Work out the finished part from the listing and answer in its coordinate system (mm). A direction names the side the tool comes from. Coordinates: 2 decimals unless noted, no trailing zeros. Write each loop counter-clockwise with the first axis right and the second up, starting at its lowest first coordinate (ties: lowest second). Pieces come first, ordered by that corner, then holes. Notation, with made-up numbers: M 54,-32.75 L 106,-32.75 A35 ccw 106,5.25 Z; hole C -27.5,33 d8. An arc over 180 degrees is marked long. Answer as CSV lines item,"result". Start each with the question number.
(1) For faces 4 (the cylindrical face through (13.62, 2.46, 12.06)), 5 (the flat face through (-40, 2, 1)), determine the directions among +Z, -Z, +X, -X, +Y, -Y from which every point of the face is accessible in a straight line to the end or side of a thin tool.
(2) A flat-ended cylindrical pin translates along its axis: P1, Ø2.5, axis at x = 25, z = -34, coming from the -Y side. Find the tip coordinate at first contact, or state that the pin passes through.
(3) Find the intervals of material crossed by L1, parallel to Z at x = 25, y = 3.25; L2, parallel to X at y = 3.1, z = 34; L3, parallel to Z at x = -4, y = 3.7, in increasing order. Write a range as [from, to].
(4) A cutting plane is placed at C-C on y = 2.6. Give the vertices of the cut face in (x, z).
(5) The mould has two halves that part along Z. Classify faces 1 (the flat face through (-5, 2, 39)), 2 (the flat face through (-5, 2, 13.621)), 3 (the cylindrical face through (-39.14, 2.54, -38.1)): released by +Z, released by -Z, zero draft, split by the parting line, or undercut.
(6) A cutting plane is placed at D-D on x = -7. Give the vertices of the cut face in (y, z), then the cut area to 3 significant figures.
(7) A cutting plane is placed at B-B on z = 0. Give the vertices of the cut face in (x, y), then the cut area to 3 significant figures.
(8) A cutting plane is placed at A-A on x = 25. Give the vertices of the cut face in (y, z), then the cut area to 3 significant figures.
from build123d import *

# Parameters (mm, degrees)
SKETCH1_W           = 70
SKETCH1_H           = 78
SKETCH1_R           = 2.25
BOSS_EXTRUDE1_DEPTH = 5
FILLET1_R           = 3


with BuildPart() as part:
    # Sketch1 → Boss-Extrude1 (new body)
    with BuildSketch(Plane(origin=(0, 0, 0), x_dir=(1, 0, 0), z_dir=(0, 1, 0))):
        with Locations((-5, 0)):
            Rectangle(SKETCH1_W, SKETCH1_H)
        with Locations((-35, 34)):
            Circle(SKETCH1_R, mode=Mode.SUBTRACT)
        with Locations((25, 34)):
            Circle(SKETCH1_R, mode=Mode.SUBTRACT)
        with Locations((25, -34)):
            Circle(SKETCH1_R, mode=Mode.SUBTRACT)
        with Locations((-35, -34)):
            Circle(SKETCH1_R, mode=Mode.SUBTRACT)
        with BuildLine():
            Line((-22.02081528, 13.62081528), (12.02081528, 13.62081528))
            ThreePointArc((12.02081528, 13.62081528), (13.62081528, 12.02081528), (12.02081528, 10.42081528))
            Line((12.02081528, 10.42081528), (-22.02081528, 10.42081528))
            ThreePointArc((-22.02081528, 10.42081528), (-23.62081528, 12.02081528), (-22.02081528, 13.62081528))
        make_face(mode=Mode.SUBTRACT)
        with BuildLine():
            Line((-22.02081528, -13.62081528), (12.02081528, -13.62081528))
            ThreePointArc((12.02081528, -13.62081528), (13.62081528, -12.02081528), (12.02081528, -10.42081528))
            Line((12.02081528, -10.42081528), (-22.02081528, -10.42081528))
            ThreePointArc((-22.02081528, -10.42081528), (-23.62081528, -12.02081528), (-22.02081528, -13.62081528))
        make_face(mode=Mode.SUBTRACT)
        with BuildLine():
            Line((-10, 5), (0, 5))
            ThreePointArc((0, 5), (5, 0), (0, -5))
            Line((0, -5), (-10, -5))
            ThreePointArc((-10, -5), (-15, 0), (-10, 5))
        make_face(mode=Mode.SUBTRACT)
    extrude(amount=BOSS_EXTRUDE1_DEPTH)

    # Fillet1
    fillet1_edges = [part.edges().sort_by_distance(p)[0] for p in [
        (30, 2.5, -39),
        (30, 2.5, 39),
        (-40, 2.5, 39),
        (-40, 2.5, -39),
    ]]
    fillet(fillet1_edges, radius=FILLET1_R)


solid = part.part
Here are the results:
1,face 4,"+Y, -Y"
1,face 5,"+Z, -Z, -X, +Y, -Y"
2,P1,"passes through"
3,L1,"z = [-39, -36.25], [-31.75, 31.75], [36.25, 39]"
3,L2,"x = [-40, -37.25], [-32.75, 22.75], [27.25, 30]"
3,L3,"z = [-39, -13.62], [-10.42, -5], [5, 10.42], [13.62, 39]"
4,outline,"M -40,-36 A3 ccw -37,-39 L 27,-39 A3 ccw 30,-36 L 30,36 A3 ccw 27,39 L -37,39 A3 ccw -40,36 Z; hole C -35,-34 d4.5; hole C -35,34 d4.5; hole M -22.02,-13.62 L 12.02,-13.62 A1.6 ccw 12.02,-10.42 L -22.02,-10.42 A1.6 ccw Z; hole M -22.02,10.42 L 12.02,10.42 A1.6 ccw 12.02,13.62 L -22.02,13.62 A1.6 ccw Z; hole M -10,-5 L 0,-5 A5 ccw 0,5 L -10,5 A5 ccw Z; hole C 25,-34 d4.5; hole C 25,34 d4.5"
5,face 1,"released by +Z"
5,face 2,"undercut"
5,face 3,"released by -Z"
6,outline,"M 0,-39 L 5,-39 L 5,-13.62 L 0,-13.62 Z; M 0,-10.42 L 5,-10.42 L 5,-5 L 0,-5 Z; M 0,5 L 5,5 L 5,10.42 L 0,10.42 Z; M 0,13.62 L 5,13.62 L 5,39 L 0,39 Z"
6,area,"308 mm^2"
7,outline,"M -40,0 L -15,0 L -15,5 L -40,5 Z; M 5,0 L 30,0 L 30,5 L 5,5 Z"
7,area,"250 mm^2"
8,outline,"M 0,-39 L 5,-39 L 5,-36.25 L 0,-36.25 Z; M 0,-31.75 L 5,-31.75 L 5,31.75 L 0,31.75 Z; M 0,36.25 L 5,36.25 L 5,39 L 0,39 Z"
8,area,"345 mm^2"
